from build123d import *

# Parameters (mm, degrees)
SKETCH1_R           = 2.4
BOSS_EXTRUDE1_DEPTH = 110


with BuildPart() as part:
    # Sketch1 → Boss-Extrude1 (new body)
    with BuildSketch(Plane(origin=(0, 0, 0), x_dir=(1, 0, 0), z_dir=(0, 1, 0))):
        with BuildLine():
            ThreePointArc((-10, -9), (-9.707106781, -9.707106781), (-9, -10))
            Line((-9, -10), (-3.1, -10))
            Line((-3.1, -10), (-3.1, -8.7))
            ThreePointArc((-3.1, -8.7), (-3.246446609, -8.346446609), (-3.6, -8.2))
            Line((-3.6, -8.2), (-5.5, -8.2))
            Line((-5.5, -8.2), (-5.5, -6.376528763))
            Line((-5.5, -6.376528763), (-3.123471237, -4))
            Line((-3.123471237, -4), (0, -4))
            Line((0, -4), (3.123471237, -4))
            Line((3.123471237, -4), (5.5, -6.376528763))
            Line((5.5, -6.376528763), (5.5, -8.2))
            Line((5.5, -8.2), (3.6, -8.2))
            ThreePointArc((3.6, -8.2), (3.246446609, -8.346446609), (3.1, -8.7))
            Line((3.1, -8.7), (3.1, -10))
            Line((3.1, -10), (9, -10))
            ThreePointArc((9, -10), (9.707106781, -9.707106781), (10, -9))
            Line((10, -9), (10, -3.1))
            Line((10, -3.1), (8.7, -3.1))
            ThreePointArc((8.7, -3.1), (8.346446609, -3.246446609), (8.2, -3.6))
            Line((8.2, -3.6), (8.2, -5.5))
            Line((8.2, -5.5), (6.376528763, -5.5))
            Line((6.376528763, -5.5), (4, -3.123471237))
            Line((4, -3.123471237), (4, 0))
            Line((4, 0), (4, 3.123471237))
            Line((4, 3.123471237), (6.376528763, 5.5))
            Line((6.376528763, 5.5), (8.2, 5.5))
            Line((8.2, 5.5), (8.2, 3.6))
            ThreePointArc((8.2, 3.6), (8.346446609, 3.246446609), (8.7, 3.1))
            Line((8.7, 3.1), (10, 3.1))
            Line((10, 3.1), (10, 9))
            ThreePointArc((10, 9), (9.707106781, 9.707106781), (9, 10))
            Line((9, 10), (3.1, 10))
            Line((3.1, 10), (3.1, 8.7))
            ThreePointArc((3.1, 8.7), (3.246446609, 8.346446609), (3.6, 8.2))
            Line((3.6, 8.2), (5.5, 8.2))
            Line((5.5, 8.2), (5.5, 6.376528763))
            Line((5.5, 6.376528763), (3.123471237, 4))
            Line((3.123471237, 4), (0, 4))
            Line((0, 4), (-3.123471237, 4))
            Line((-3.123471237, 4), (-5.5, 6.376528763))
            Line((-5.5, 6.376528763), (-5.5, 8.2))
            Line((-5.5, 8.2), (-3.6, 8.2))
            ThreePointArc((-3.6, 8.2), (-3.246446609, 8.346446609), (-3.1, 8.7))
            Line((-3.1, 8.7), (-3.1, 10))
            Line((-3.1, 10), (-9, 10))
            ThreePointArc((-9, 10), (-9.707106781, 9.707106781), (-10, 9))
            Line((-10, 9), (-10, 3.1))
            Line((-10, 3.1), (-8.7, 3.1))
            ThreePointArc((-8.7, 3.1), (-8.346446609, 3.246446609), (-8.2, 3.6))
            Line((-8.2, 3.6), (-8.2, 5.5))
            Line((-8.2, 5.5), (-6.376528763, 5.5))
            Line((-6.376528763, 5.5), (-4, 3.123471237))
            Line((-4, 3.123471237), (-4, 0))
            Line((-4, 0), (-4, -3.123471237))
            Line((-4, -3.123471237), (-6.376528763, -5.5))
            Line((-6.376528763, -5.5), (-8.2, -5.5))
            Line((-8.2, -5.5), (-8.2, -3.6))
            ThreePointArc((-8.2, -3.6), (-8.346446609, -3.246446609), (-8.7, -3.1))
            Line((-8.7, -3.1), (-10, -3.1))
            Line((-10, -3.1), (-10, -9))
        make_face()
        Circle(SKETCH1_R, mode=Mode.SUBTRACT)
    extrude(amount=BOSS_EXTRUDE1_DEPTH)


solid = part.part
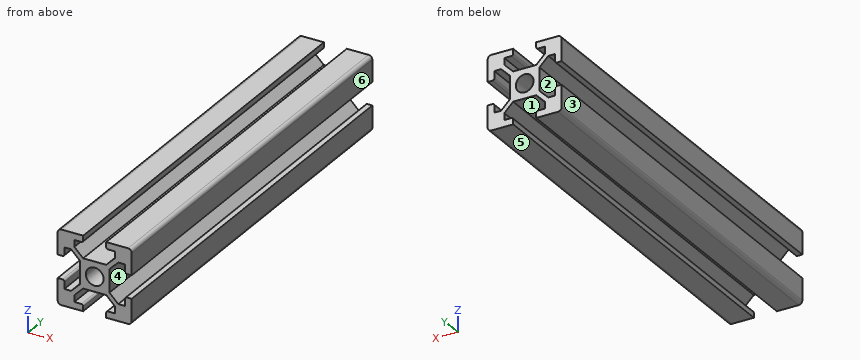
The listing builds one solid part. Answer for the finished solid, in the listing's coordinates (mm). Face numbers are marked on the shaded views. A direction names the side the tool comes from. Give positions to 0.01 mm unless a question says otherwise; leave off trailing zeros. Write each loop counter-clockwise with the first axis right and the second up, starting at its lowest first coordinate (ties: lowest second). Pieces come first, ordered by that corner, then holes.
1) For a pull along Z with two mould halves and no side action, classify the marked faces 4, 5 and 6 as pulls with the +Z half, pulls with the -Z half, needs draft (parallel to the pull), parting line crosses it, or undercut.
2) Find the intervals of material crossed by L1, parallel to Z at x = 0, y = 30; L2, parallel to Z at x = -6.5, y = 38, in increasing order.
3) A tool of negligible diameter and unlimited length cuts with its end or side. For the marked faces 1, 2 and 3, from which of +Z, -Z, +X, -X, +Y, -Y can it reach the whole face along a straight path? Write none if from no direction.
4) Given P1, Ø2, axis at x = -2, y = 51.5, coming from the +Z side; P2, Ø4.5, axis at x = 0, z = 0, coming from the +Y side; P3, Ø0.7, axis at x = 9.5, y = 74, coming from the +Z side, each flat-ended and moving along its own axis, determine where each tip first touches the part or whether it passes through.
5) Section B-B (x = 0) is taken. Write down the section's boundary in (y, z).
6) Section A-A (z = 0) is taken. Write down the section's boundary in (x, y).
Response:
1. face 4: undercut
1. face 5: pulls with the -Z half
1. face 6: needs draft
2. L1: z = -4 to -2.4, 2.4 to 4
2. L2: z = -10 to -5.5, 5.5 to 10
3. face 1: -Z, +Y, -Y
3. face 2: -X, +Y, -Y
3. face 3: +Z, -Z, -X, +Y, -Y
4. P1: stops at z = 4
4. P2: passes through
4. P3: stops at z = 9.99
5. outline: (0, -4) - (110, -4) - (110, -2.4) - (0, -2.4) - close; (0, 2.4) - (110, 2.4) - (110, 4) - (0, 4) - close
6. outline: (-4, 0) - (-2.4, 0) - (-2.4, 110) - (-4, 110) - close; (2.4, 0) - (4, 0) - (4, 110) - (2.4, 110) - close
